Source: CAD feature listing. Evaluate the final solid. Frame: model axes, mm. A direction names the side the tool comes from. Give positions to 0.01 mm unless a question says otherwise; leave off trailing zeros. Order: outer loops, then holes, each group sorted by start corner. A loop starts at its lowest first (then second) coordinate and runs counter-clockwise, first axis right, second up.
from build123d import *

# Parameters (mm, degrees)
SKETCH1_W                = 31.75
SKETCH1_H                = 14.2875
REVOLVE1_ANGLE           = 358
CUT_EXTRUDE1_DEPTH       = 55.99261314
CUT_EXTRUDE2_START       = -25.4
CUT_EXTRUDE2_DEPTH       = 25.4
DRAFT1_ANGLE             = 1.79
M7_CLEARANCE_HOLE1_D     = 7.62
M7_CLEARANCE_HOLE1_DEPTH = 31.75
HOLE1_D                  = 6.35
HOLE1_DEPTH              = 31.75


with BuildPart() as part:
    # Sketch1 → Revolve1 (revolve)
    with BuildSketch(Plane(origin=(0, 0, 0), x_dir=(1, 0, 0), z_dir=(0, -0.017452406437279848, -0.9998476951563914))):
        with Locations((9.525, 24.60625)):
            Rectangle(SKETCH1_W, SKETCH1_H)
    revolve(axis=Axis((-6.35, 0, 0), (-1, 0, 0)), revolution_arc=REVOLVE1_ANGLE)

    # Sketch2 → Cut-Extrude1 (cut, through all)
    with BuildSketch(Plane.ZY.offset(6.35)):
        with BuildLine():
            Line((3.96875, 17.005526445), (3.96875, 19.05))
            Line((3.96875, 19.05), (-3.96875, 19.05))
            Line((-3.96875, 19.05), (-3.96875, 17.005526445))
            ThreePointArc((-3.96875, 17.005526445), (0, 17.4625), (3.96875, 17.005526445))
        make_face()
    extrude(amount=-CUT_EXTRUDE1_DEPTH, mode=Mode.SUBTRACT)

    # Sketch3 → Cut-Extrude2 (cut)
    with BuildSketch(Plane(origin=(25.4, 0, 0), x_dir=(0, 0, -1), z_dir=(1, 0, 0)).offset(CUT_EXTRUDE2_START)):
        with BuildLine():
            Line((0.360174038, -20.634356809), (0.554113904, -31.745164321))
            ThreePointArc((0.554113904, -31.745164321), (0, 31.75), (-0.554113904, -31.745164321))
            Line((-0.554113904, -31.745164321), (-0.360174038, -20.634356809))
            ThreePointArc((-0.360174038, -20.634356809), (0, 20.6375), (0.360174038, -20.634356809))
        make_face()
    extrude(amount=CUT_EXTRUDE2_DEPTH, mode=Mode.SUBTRACT)

    # Draft1
    draft1_faces = [part.faces().sort_by_distance(p)[0] for p in [
        (12.7, 20.6375, 0),
    ]]
    draft(draft1_faces, Plane(origin=(0, 0, 0), x_dir=(0, 0, 1), z_dir=(1, 0, 0)), DRAFT1_ANGLE)

    # M7 Clearance Hole1
    with Locations(Plane.ZY.offset(6.35)):
        with Locations((-17.823234059, -18.096749091), (17.823234059, 18.096749091)):
            Hole(M7_CLEARANCE_HOLE1_D / 2, depth=M7_CLEARANCE_HOLE1_DEPTH)

    # Hole1
    with Locations(Plane.ZY.offset(6.35)):
        with Locations((-17.823234059, 18.096749091), (17.823234059, -18.096749091)):
            Hole(HOLE1_D / 2, depth=HOLE1_DEPTH)


solid = part.part
1) Reachability of faces 4 (the face through (9, 18, 3.969)), 5 (the face through (-6.35, 13, -14)), 6 (the face through (0, 0, -21)) from +Z, -Z, +X, -X, +Y, -Y: full face, straight path, thin tool, end or side. Return the list, or none.
Checks:
face 4: +X, -X
face 5: +Z, -Z, -X, +Y, -Y
face 6: +X
2) Ray query, L1, parallel to X at y = -22, z = -14.5; L2, parallel to Y at x = 16, z = 4; L3, parallel to Z at x = 24.5, y = -14. Return the intervals inside material, ascending.
Checks:
L1: x = -6.35 to 0
L2: y = -19.74 to -17, 17 to 19.74
L3: z = -14.1 to -10.44, 10.44 to 14.1
3) Section query B-B on x = -2.5. State how many separate pieces and enclosed holes the cut face has, and give its area (3 significant figures).
Checks:
separate pieces: 1
enclosed holes: 4
area: 2,030 mm2
4) Section query A-A on y = 0. Output: boundary loops of the cut face in (x, z).
Checks:
outline: (-6.35, -31.75) - (0, -31.75) - (0, -20.64) - (25.4, -19.84) - (25.4, -17.46) - (-6.35, -17.46) - close; (-6.35, 17.46) - (25.4, 17.46) - (25.4, 19.84) - (0, 20.64) - (0, 31.75) - (-6.35, 31.75) - close
5) Section query D-D on z = -23. Output: boundary loops of the cut face in (x, y).
Checks:
outline: (-6.35, -21.89) - (0, -21.89) - (0, 21.89) - (-6.35, 21.89) - close
6) First-contact query: pin 1 Ø2 at (y, z) = (11.5, 25.5) entering from +X; pin 2 Ø10 at (x, z) = (11.5, -22.5) entering from -Y; pin 3 Ø6.5 at (x, z) = (14, 0) entering from -Y; pin 4 Ø5.5 at (y, z) = (-18.1, 17.82) entering from -X. Flat tips, straight axial feed; report the tip coordinate or a pass-through.
Checks:
pin 1: stops at x = 0
pin 2: stops at y = -10.25
pin 3: stops at y = -20.3
pin 4: passes through
7) Pull-direction query (Y, two-part tool) for faces 1 (the face through (12.522, 20.227, 0.885)), 2 (the face through (9, 18, -3.969)), 3 (the face through (25.4, -14, -11)); classes: +Y half, -Y half, draft (parallel to the pull), parting line (faces both ways), or undercut.
Checks:
face 1: parting line
face 2: undercut
face 3: draft
